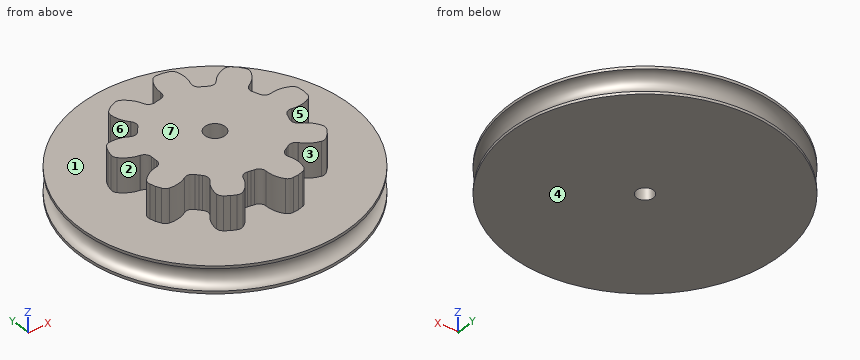
from build123d import *

# Parameters (mm, degrees)
F1_DEPTH = 5
F2_COUNT = 9
F4_R     = 1.5
F5_DEPTH = 5


with BuildPart() as f1:
    # F0 (on Top) → F1 (new body)
    with BuildSketch(Plane.XY):
        with BuildLine():
            Line((8.305078, 3.467805), (0, 0))
            Line((0, 0), (8.305078, -3.467805))
            ThreePointArc((8.305078, -3.467805), (8.464361, -3.058527), (8.603489, -2.641966))
            ThreePointArc((8.603489, -2.641966), (9.047406, -2.076548), (9.755918, -1.955011))
            Line((9.755918, -1.955011), (9.805066, -1.96486))
            ThreePointArc((9.805066, -1.96486), (11.163417, -2.001728), (12.455768, -1.581844))
            ThreePointArc((12.455768, -1.581844), (12.819329, -1.255462), (12.98487, -0.795791))
            Line((12.98487, -0.795791), (13.06382, 0))
            Line((13.06382, 0), (12.98487, 0.795791))
            ThreePointArc((12.98487, 0.795791), (12.819329, 1.255462), (12.455768, 1.581844))
            ThreePointArc((12.455768, 1.581844), (11.163417, 2.001728), (9.805066, 1.96486))
            Line((9.805066, 1.96486), (9.755918, 1.955011))
            ThreePointArc((9.755918, 1.955011), (9.047406, 2.076548), (8.603489, 2.641966))
            ThreePointArc((8.603489, 2.641966), (8.464361, 3.058527), (8.305078, 3.467805))
        make_face()
    extrude(amount=F1_DEPTH)


with BuildPart() as f2_1:
    # F2: instance of F1
    add(f1.part.rotate(Axis((0, 0, 2.5), (0, 0, 1)), 1 * 360 / F2_COUNT))


with BuildPart() as f2_2:
    # F2: instance of F1
    add(f1.part.rotate(Axis((0, 0, 2.5), (0, 0, 1)), 2 * 360 / F2_COUNT))


with BuildPart() as f2_3:
    # F2: instance of F1
    add(f1.part.rotate(Axis((0, 0, 2.5), (0, 0, 1)), 3 * 360 / F2_COUNT))


with BuildPart() as f2_4:
    # F2: instance of F1
    add(f1.part.rotate(Axis((0, 0, 2.5), (0, 0, 1)), 4 * 360 / F2_COUNT))


with BuildPart() as f2_5:
    # F2: instance of F1
    add(f1.part.rotate(Axis((0, 0, 2.5), (0, 0, 1)), 5 * 360 / F2_COUNT))


with BuildPart() as f2_6:
    # F2: instance of F1
    add(f1.part.rotate(Axis((0, 0, 2.5), (0, 0, 1)), 6 * 360 / F2_COUNT))


with BuildPart() as f2_7:
    # F2: instance of F1
    add(f1.part.rotate(Axis((0, 0, 2.5), (0, 0, 1)), 7 * 360 / F2_COUNT))


with BuildPart() as f2_8:
    # F2: instance of F1
    add(f1.part.rotate(Axis((0, 0, 2.5), (0, 0, 1)), 8 * 360 / F2_COUNT))


with BuildPart() as f2_7_1:
    add(f2_7.part)

    # F3: union F2_6, F2_4, F2_5, F1, F2_1, F2_3, F2_2, F2_8
    add(f2_6.part)
    add(f2_4.part)
    add(f2_5.part)
    add(f1.part)
    add(f2_1.part)
    add(f2_3.part)
    add(f2_2.part)
    add(f2_8.part)

    # F4 (on face) → F5 (cut, through all)
    with BuildSketch(Plane.XY.offset(5)):
        Circle(F4_R)
    extrude(amount=-F5_DEPTH, mode=Mode.SUBTRACT)

    # F6 (on Right) → F7 (revolve)
    with BuildSketch(Plane.YZ):
        with BuildLine():
            Line((20, 0), (1.25, 0))
            Line((1.25, 0), (1.25, -4))
            Line((1.25, -4), (20, -4))
            Line((20, -4), (20, -3.6))
            ThreePointArc((20, -3.6), (18.4, -2), (20, -0.4))
            Line((20, -0.4), (20, 0))
        make_face()
    revolve(axis=Axis((0, 0, -1.51735), (0, 0, -1)))


solid = f2_7_1.part
Geometry check sheet. Reference: the model listing, model coordinates, mm. Face numbers are marked on the shaded views. A direction names the side the tool comes from. Give positions to 0.01 mm unless a question says otherwise; leave off trailing zeros. Order: outer loops, then holes, each group sorted by start corner. A loop starts at its lowest first (then second) coordinate and runs counter-clockwise, first axis right, second up.
1. Draft check along X on the marked faces 5, 6 and 7. Enter one of: pulls with the +X half, pulls with the -X half, needs draft (parallel to the pull), parting line crosses it, or undercut.
Completed:
face 5: undercut
face 6: pulls with the -X half
face 7: needs draft
2. Access from +Z, -Z, +X, -X, +Y, -Y to the whole of each face (thin tool, end or side, straight path). Record for the marked faces 1, 2, 3 and 4.
Completed:
face 1: +Z
face 2: +Z, -X
face 3: +Z, -Y
face 4: -Z, +X, -X, +Y, -Y
3. Depth check by flat-ended pin: pin 1 (3.5 mm diameter, centred on x = 0, y = 0, fed in from -Z); pin 2 (0.9 mm diameter, centred on x = 0, y = 0.5, fed in from +Z); pin 3 (5 mm diameter, centred on y = 12.5, z = 1, fed in from +X); pin 4 (4 mm diameter, centred on y = 2.5, z = 0, fed in from -X). Enter the tip coordinate at first touch or a pass-through.
Completed:
pin 1: stops at z = -4
pin 2: passes through
pin 3: stops at x = 17.2
pin 4: stops at x = -19.99
4. Scan lines: line 1 (Y direction, x = 9.5, z = 1.5); line 2 (Z direction, x = 5, y = -10.5); line 3 (X direction, y = 11.5, z = 0.5). Record each from-to range of solid material in increasing order.
Completed:
line 1: y = -8.89 to -5.31, -1.94 to 1.94, 5.31 to 8.89
line 2: z = -4 to 0
line 3: x = -6.12 to -4.74, 0.02 to 3.84
5. Sectioned sample at A-A (z = -2). Record the boundary of the cut face in (x, y).
Completed:
outline: circle Ø36.8 at (0, 0); hole circle Ø2.5 at (0, 0)
